The model under review builds one solid part; all positions refer to its coordinate system, in mm. Give positions to 0.01 mm unless a question says otherwise; leave off trailing zeros. Loops run counter-clockwise (first coordinate to the right, second up) from the corner with the lowest first, then second, coordinate; pieces in that order, holes last. Notation, with made-up numbers: (-1, -18.5) - (44, -18.5) arc R29 ccw to (44, 11.5) - close; hole circle Ø8 at (83, -12). An arc over 180 degrees is marked (long way). Answer as a JSON object with one key per item and string values.
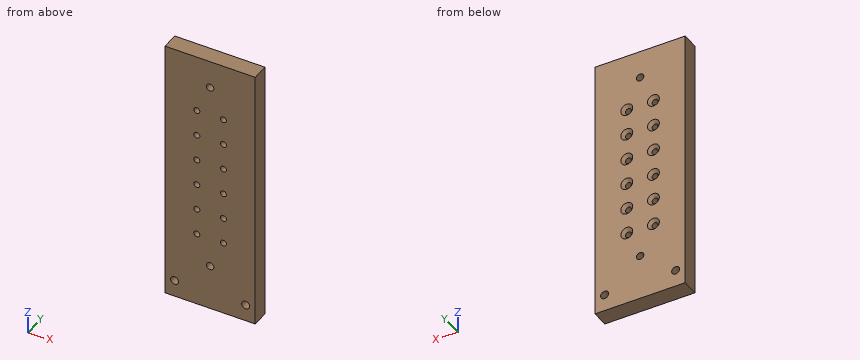
from build123d import *

# Parameters (mm, degrees)
SKETCH1_W                     = 50.8
SKETCH1_H                     = 9.525
BOSS_EXTRUDE1_DEPTH           = 75
TAP_DRILL_FOR_M5X0_8_TAP1_D   = 4.2
M4_CLEARANCE_HOLE1_D          = 4.5
CSK_FOR_M3_SFHCS1_D           = 3.4
CSK_FOR_M3_SFHCS1_CSINK_D     = 6.72
CSK_FOR_M3_SFHCS1_CSINK_ANGLE = 90
LPATTERN1_COUNT               = 6
LPATTERN1_PITCH               = 15


with BuildPart() as part:
    # Sketch1 → Boss-Extrude1 (new, symmetric)
    with BuildSketch(Plane.XY):
        Rectangle(SKETCH1_W, SKETCH1_H)
    extrude(amount=BOSS_EXTRUDE1_DEPTH, both=True)

    # Tap Drill for M5x0.8 Tap1 (through all)
    with Locations(Plane(origin=(0, 4.7625, 0), x_dir=(1, 0, 0), z_dir=(0, 1, 0))):
        with Locations((0, -59.3), (0, 49.3)):
            Hole(TAP_DRILL_FOR_M5X0_8_TAP1_D / 2)

    # M4 Clearance Hole1 (through all)
    with Locations(Plane(origin=(0, 4.7625, 0), x_dir=(1, 0, 0), z_dir=(0, 1, 0))):
        with Locations((-20, 65.475), (20, 65.475)):
            Hole(M4_CLEARANCE_HOLE1_D / 2)

    # CSK for M3 SFHCS1 (through all)
    with Locations(Plane(origin=(0, 4.7625, 0), x_dir=(1, 0, 0), z_dir=(0, 1, 0))):
        with Locations((7.5, 32.5), (-7.5, 32.5)):
            csk_for_m3_sfhcs1 = CounterSinkHole(CSK_FOR_M3_SFHCS1_D / 2, CSK_FOR_M3_SFHCS1_CSINK_D / 2, counter_sink_angle=CSK_FOR_M3_SFHCS1_CSINK_ANGLE)

    # LPattern1: CSK for M3 SFHCS1 ×6
    with Locations(*[(0, 0, i * LPATTERN1_PITCH) for i in range(1, LPATTERN1_COUNT)]):
        add(csk_for_m3_sfhcs1, mode=Mode.SUBTRACT)


solid = part.part
Q1. Consider section B-B, the plane x = 0. State the section outline as (y, z) points.
Results:
{"outline": "(-4.76, -75) - (4.76, -75) - (4.76, -51.4) - (-4.76, -51.4) - close; (-4.76, -47.2) - (4.76, -47.2) - (4.76, 57.2) - (-4.76, 57.2) - close; (-4.76, 61.4) - (4.76, 61.4) - (4.76, 75) - (-4.76, 75) - close"}
Q2. Clearance check with flat-ended pins moving along their axes: pin 1 Ø3 at (x, z) = (-7.5, 12.5) entering from -Y; pin 2 Ø5.5 at (x, z) = (7.5, 27.5) entering from +Y; pin 3 Ø4.5 at (x, z) = (-7.5, -17.5) entering from +Y. State where each tip first meets the part, or that it passes through.
Results:
{"pin 1": "passes through", "pin 2": "stops at y = 4.15", "pin 3": "stops at y = 3.65"}
Q3. Consider section C-C, the plane z = -49.3. State the section outline as (x, y) points.
Results:
{"outline": "(-25.4, -4.76) - (-2.1, -4.76) - (-2.1, 4.76) - (-25.4, 4.76) - close; (2.1, -4.76) - (25.4, -4.76) - (25.4, 4.76) - (2.1, 4.76) - close"}
Q4. Consider section D-D, the plane x = 20. State the section outline as (y, z) points (1 decimal).
Results:
{"outline": "(-4.8, -75) - (4.8, -75) - (4.8, -67.7) - (-4.8, -67.7) - close; (-4.8, -63.2) - (4.8, -63.2) - (4.8, 75) - (-4.8, 75) - close"}
Q5. To check wall thickness, follow probe 1 along X at (y, z) = (0.5, -17.5); probe 2 along Z at (x, y) = (0, -1); probe 3 along X at (y, z) = (1.5, -49.3). State the ranges of each line that lie inside material, in increasing order. Write a range as [from, to].
Results:
{"probe 1": "x = [-25.4, -9.2], [-5.8, 5.8], [9.2, 25.4]", "probe 2": "z = [-75, -51.4], [-47.2, 57.2], [61.4, 75]", "probe 3": "x = [-25.4, -2.1], [2.1, 25.4]"}
Q6. Consider section A-A, the plane z = 27.5. State the section outline as (x, y) points.
Results:
{"outline": "(-25.4, -4.76) - (-9.2, -4.76) - (-9.2, 3.1) - (-10.86, 4.76) - (-25.4, 4.76) - close; (-5.8, -4.76) - (5.8, -4.76) - (5.8, 3.1) - (4.14, 4.76) - (-4.14, 4.76) - (-5.8, 3.1) - close; (9.2, -4.76) - (25.4, -4.76) - (25.4, 4.76) - (10.86, 4.76) - (9.2, 3.1) - close"}
